For this review, take the finished solid that the model builds, in its own axes (mm). Face numbers are marked on the shaded views. A direction names the side the tool comes from. Round coordinates to 2 decimals unless told otherwise and drop trailing zeros. Order: outer loops, then holes, each group sorted by start corner. A loop starts at its lowest first (then second) coordinate and runs counter-clockwise, first axis right, second up.
from build123d import *

# Parameters (mm, degrees)
CHAMFER1_SIZE = 1


with BuildPart() as part:
    # Sketch1 → Revolve1 (revolve)
    with BuildSketch(Plane.XY, mode=Mode.PRIVATE) as revolve1_sk:
        Polygon((7, 0), (7, 14), (10, 14), (10, 12), (9, 12), (9, 2), (10, 2), (10, 0), align=None)
    revolve(revolve1_sk.sketch.rotate(Axis((0, 0.1, 0), (0, 1, 0)), 90), axis=Axis((0, 0.1, 0), (0, 1, 0)))

    # Chamfer1
    chamfer1_edges = [part.edges().sort_by_distance(p)[0] for p in [
        (0, 12, 9),
    ]]
    chamfer(chamfer1_edges, length=CHAMFER1_SIZE - 0.0001)  # a hair under: the kernel refuses the full size


solid = part.part
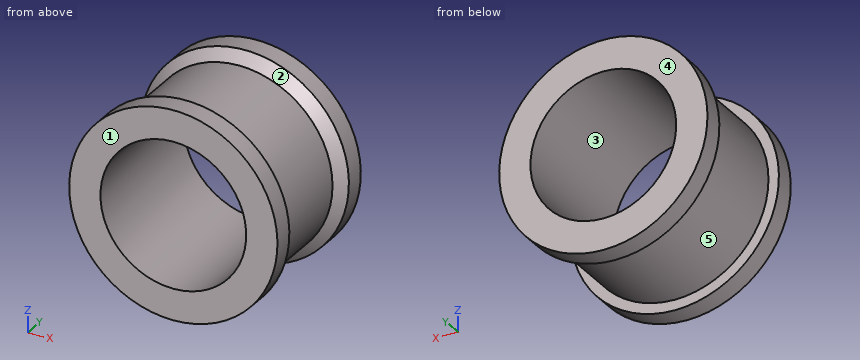
(1) Wall thickness on L1, parallel to X at y = 6.75, z = 0; L2, parallel to X at y = 9, z = 5.5; L3, parallel to Z at x = 6, y = 13: over which ranges is each line inside the solid? List them lowest first.
(2) Tool access review of the marked faces 1 and 2: name each direction out of +Z, -Z, +X, -X, +Y, -Y from which nothing blocks a thin tool from reaching the whole face with its end or side.
(3) Add section D-D on y = 1.5. Give the boundary of the cut face in (x, z).
(4) Draft analysis for pull direction Z (two halves, no side actions). For the marked faces 3, 4 and 5, state which applies: pulls with the +Z half, pulls with the -Z half, needs draft (parallel to the pull), parting line crosses it, or undercut.
(5) Clearance check with flat-ended pins moving along their axes: P1, Ø3, axis at x = 6, y = 10.5, coming from the -Z side; P2, Ø3, axis at x = 2, y = 10.5, coming from the +Z side; P3, Ø11, axis at x = 0, z = 0, coming from the -Y side; P4, Ø6, axis at y = 1.5, z = -7.5, coming from the +X side. State where each tip first meets the part, or that it passes through.
(6) Add section C-C on y = 5.25. Give the boundary of the cut face in (x, z).
Here are the results:
1. L1: x = -9 to -7, 7 to 9
1. L2: x = -7.12 to -4.33, 4.33 to 7.12
1. L3: z = -8 to -3.61, 3.61 to 8
2. face 1: +Z, -Z, +X, -X, -Y
2. face 2: none
3. outline: circle Ø20 at (0, 0); hole circle Ø14 at (0, 0)
4. face 3: undercut
4. face 4: needs draft
4. face 5: parting line crosses it
5. P1: stops at z = -8.27
5. P2: stops at z = 9.82
5. P3: passes through
5. P4: stops at x = 8.93
6. outline: circle Ø18 at (0, 0); hole circle Ø14 at (0, 0)
